from build123d import *

# Parameters (mm, degrees)
SKETCH1_R                = 1.5
BOSS_EXTRUDE1_DEPTH      = 40
BOSS_EXTRUDE2_DEPTH      = 1.5
BOSS_EXTRUDE2_DEPTH_BACK = 1.5
SKETCH6_W                = 4.5
SKETCH6_H                = 13
CUT_EXTRUDE2_DEPTH       = 4
SKETCH13_R               = 1.5
BOSS_EXTRUDE3_DEPTH      = 30


with BuildPart() as part:
    # Sketch1 → Boss-Extrude1 (new body)
    with BuildSketch(Plane(origin=(0, 0, 0), x_dir=(1, 0, 0), z_dir=(0, 1, 0))):
        with Locations(Location((0, 0, 0), (0, 0, 270))):
            Circle(SKETCH1_R)
    extrude(amount=BOSS_EXTRUDE1_DEPTH)

    # Sketch6 → Boss-Extrude2 (add, two sides: drawn at the far end of the back side and taken through both)
    with BuildSketch(Plane.XY.offset(-BOSS_EXTRUDE2_DEPTH_BACK)):
        with Locations((0.75, 33.5)):
            Rectangle(SKETCH6_W, SKETCH6_H)
    extrude(amount=BOSS_EXTRUDE2_DEPTH + BOSS_EXTRUDE2_DEPTH_BACK)

    # Sketch12 → Cut-Extrude2 (cut)
    with BuildSketch(Plane.XY.offset(1.5)):
        Polygon((3, 40), (3, 37), (0.5, 38.010065565), (0.5, 38.989934435), align=None)
        Polygon((0.5, 34.369934435), (0.5, 33.390065565), (3, 32.38), (3, 35.38), align=None)
        Polygon((0.5, 29.749934435), (0.5, 28.770065565), (3, 27.76), (3, 30.76), align=None)
    extrude(amount=-CUT_EXTRUDE2_DEPTH, mode=Mode.SUBTRACT)

    # Sketch13 → Boss-Extrude3 (add)
    with BuildSketch(Plane(origin=(0, 40, 0), x_dir=(1, 0, 0), z_dir=(0, 1, 0))):
        with Locations(Location((0, 0, 0), (0, 0, 270))):
            Circle(SKETCH13_R)
    extrude(amount=BOSS_EXTRUDE3_DEPTH)


solid = part.part
For this review, take the finished solid that the model builds, in its own axes (mm). A direction names the side the tool comes from. Round coordinates to 2 decimals unless told otherwise and drop trailing zeros. Loops run counter-clockwise (first coordinate to the right, second up) from the corner with the lowest first, then second, coordinate; pieces in that order, holes last. Notation, with made-up numbers: (-39, 41) - (10, 41) arc R26 ccw to (10, 69) - close; hole circle Ø11 at (62, 74). An arc over 180 degrees is marked (long way). Put each result on its own line as item: value. Start each with the question number.
1. Consider section C-C on y = 10. State the section outline as (x, z) points.
2. Insertion check: P1, Ø0.8, axis at y = 38.5, z = -0.5, coming from the +X side; P2, Ø1.1, axis at y = 29, z = 0.5, coming from the +X side. Each pin has a flat end and moves straight along its axis. Give the tip position at first contact, or say it passes through.
3. For probe 1 along Y at (x, z) = (2, 0.4); probe 2 along Y at (x, z) = (1.8, 0.05); probe 3 along Y at (x, z) = (-1.3, 1.25), list the stretches that pass through material, from the lowest coordinate up. Write a range as [from, to].
4. For faces 1 (the flat face through (2, 40, 0)), 2 (the flat face through (1.733, 28.272, 0.021)), 3 (the flat face through (-1.2, 27, -1.14)), list the 3-axis set-ups (+Z, -Z, +X, -X, +Y, -Y) from which the entire face can be reached by the end or side of a thin tool; tool diameter is ignored.
5. Mouldability with a two-part tool opening along Y and no side actions: class faces 4 (the flat face through (-1.2, 40, -1.14)), 5 (the flat face through (-1.5, 33, 0)), 6 (the flat face through (1.733, 39.488, 0.021)) as +Y half, -Y half, draft (parallel to the pull), parting line (faces both ways), or undercut.
6. Consider section B-B on x = -0.85. State the section outline as (y, z) points.
7. Consider section A-A on z = 0.55. State the section outline as (x, y) points.
Result sheet:
1. outline: circle Ø3 at (0, 0)
2. P1: x = 0.5
2. P2: x = 1.29
3. probe 1: [27, 28.16], [30.36, 32.78], [34.98, 37.4], [39.6, 40]
3. probe 2: [27, 28.24], [30.28, 32.86], [34.9, 37.48], [39.52, 40]
3. probe 3: [27, 40]
4. face 1: +X, +Y
4. face 2: +Z, -Z, +X
4. face 3: -Z, -X, -Y
5. face 4: +Y half
5. face 5: draft
5. face 6: undercut
6. outline: (0, -1.24) - (27, -1.24) - (27, -1.5) - (40, -1.5) - (40, -1.24) - (70, -1.24) - (70, 1.24) - (40, 1.24) - (40, 1.5) - (27, 1.5) - (27, 1.24) - (0, 1.24) - close
7. outline: (-1.5, 27) - (-1.4, 27) - (-1.4, 0) - (1.4, 0) - (1.4, 27) - (3, 27) - (3, 27.76) - (0.5, 28.77) - (0.5, 29.75) - (3, 30.76) - (3, 32.38) - (0.5, 33.39) - (0.5, 34.37) - (3, 35.38) - (3, 37) - (0.5, 38.01) - (0.5, 38.99) - (3, 40) - (1.4, 40) - (1.4, 70) - (-1.4, 70) - (-1.4, 40) - (-1.5, 40) - close
